Could you check a few things on this model? Use its own coordinates, in mm. A direction names the side the tool comes from. Give positions to 0.01 mm unless a question says otherwise; leave off trailing zeros. Order: outer loops, then holes, each group sorted by start corner. A loop starts at its lowest first (then second) coordinate and runs counter-clockwise, first axis right, second up. Notation, with made-up numbers: (46.25, 35) - (64.25, 35) arc R32 cw to (64.25, 70) - close; hole circle Ø2 at (64.25, -3.5). An arc over 180 degrees is marked (long way). Put each result on its own line as item: value.
from build123d import *

# Parameters (mm, degrees)
EXTRUDE_1_DEPTH = 8


with BuildPart() as part:
    # 草图1 → 凸台-拉伸1 (new body)
    with BuildSketch(Plane(origin=(0, 0, 0), x_dir=(1, 0, 0), z_dir=(0, 1, 0))):
        with BuildLine():
            Line((0, 5), (23, 5))
            ThreePointArc((23, 5), (28, 0), (23, -5))
            Line((23, -5), (0, -5))
            ThreePointArc((0, -5), (-5, 0), (0, 5))
        make_face()
    extrude(amount=EXTRUDE_1_DEPTH)

    # 草图2 → 切除-旋转1 (revolve, cut)
    with BuildSketch(Plane.XY):
        Polygon((0, 8), (-2.075, 8), (-2.075, 3.5), (-3.75, 3.5), (-3.75, 0), (0, 0), align=None)
    revolve(axis=Axis((0, 0, 0), (0, 1, 0)), mode=Mode.SUBTRACT)

    # 草图3 → 切除-旋转2 (revolve, cut)
    with BuildSketch(Plane.XY):
        Polygon((23, 8), (20.925, 8), (20.925, 3.5), (19.25, 3.5), (19.25, 0), (23, 0), align=None)
    revolve(axis=Axis((23, 0, 0), (0, 1, 0)), mode=Mode.SUBTRACT)


solid = part.part
1) I'm going to push flat-ended pins straight in: pin 1 (2 mm diameter, centred on y = 2, z = 3, fed in from -X); pin 2 (4.5 mm diameter, centred on x = 0, z = 0, fed in from -Y). Where does each tip first touch, or does it pass through?
Filled in:
pin 1: stops at x = -4.58
pin 2: stops at y = 3.5
2) If I drill on line 1 (Z direction, x = 23, y = 4.6) (3 decimals); line 2 (Z direction, x = 23, y = 1); line 3 (Y direction, x = 26, z = -1), over which ranges is the centre line in solid material (lowest first)? Write a range as [from, to].
Filled in:
line 1: z = [-5, -2.075], [2.075, 5]
line 2: z = [-5, -3.75], [3.75, 5]
line 3: y = [3.5, 8]
3) Suppose I cut it at D-D, the plane z = 3.25. List the corners of the cut face in (x, y) for me, and give its area (3 significant figures).
Filled in:
outline: (-3.8, 0) - (-1.87, 0) - (-1.87, 3.5) - (1.87, 3.5) - (1.87, 0) - (21.13, 0) - (21.13, 3.5) - (24.87, 3.5) - (24.87, 0) - (26.8, 0) - (26.8, 8) - (-3.8, 8) - close
area: 219 mm^2
4) Suppose I cut it at A-A, the plane z = 0. List the corners of the cut face in (x, y) for me (3 decimals), and give its area (3 significant figures).
Filled in:
outline: (-5, 0) - (-3.75, 0) - (-3.75, 3.5) - (-2.075, 3.5) - (-2.075, 8) - (-5, 8) - close; (2.075, 3.5) - (3.75, 3.5) - (3.75, 0) - (19.25, 0) - (19.25, 3.5) - (20.925, 3.5) - (20.925, 8) - (2.075, 8) - close; (25.075, 3.5) - (26.75, 3.5) - (26.75, 0) - (28, 0) - (28, 8) - (25.075, 8) - close
area: 174 mm^2
5) Suppose I cut it at C-C, the plane x = 20.5. List the corners of the cut face in (y, z) for me.
Filled in:
outline: (0, -5) - (8, -5) - (8, 5) - (0, 5) - (0, 2.8) - (3.5, 2.8) - (3.5, -2.8) - (0, -2.8) - close
6) We'd pull the mould along X, two halves only. Please class faces 3 (the cylindrical face through (21.02, 5.72, 0.62)), 4 (the cylindrical face through (-5, 4, 0)), 5 (the flat face through (12, 0, 0)): pulls with the +X half, pulls with the -X half, needs draft (parallel to the pull), parting line crosses it, or undercut.
Filled in:
face 3: undercut
face 4: pulls with the -X half
face 5: needs draft
7) Suppose I cut it at B-B, the plane y = 2.5. List the corners of the cut face in (x, z) for me, and give its area (3 significant figures).
Filled in:
outline: (0, -5) - (23, -5) arc R5 ccw to (23, 5) - (0, 5) arc R5 ccw to start; hole circle Ø7.5 at (0, 0); hole circle Ø7.5 at (23, 0)
area: 220 mm^2
8) Which directions (+Z, -Z, +X, -X, +Y, -Y) give clear straight access to the entire face, cutting with the end or side of a thin tool? Please do faces 1 (the flat face through (2, 3.5, -2)), 2 (the flat face through (12, 8, 0)).
Filled in:
face 1: -Y
face 2: +Z, -Z, +X, -X, +Y
